Could you check a few things on this model? Use its own coordinates, in mm. Coordinates: 2 decimals unless noted, no trailing zeros. Order: outer loops, then holes, each group sorted by start corner. A loop starts at its lowest first (then second) coordinate and runs counter-clockwise, first axis right, second up. Notation, with made-up numbers: (66, 13.5) -> (107, 13.5) arc R11 ccw to (107, 31.5) -> close; hole circle Ø4 at (-30.75, 69). An arc over 180 degrees is marked (long way). Use a Markdown table: item, result. Add a question column.
1) If I drill on L1, parallel to X at y = 2.2, z = -14; L2, parallel to X at y = 2.75, z = -11.75; L3, parallel to Z at x = -60, y = 2.85, over which ranges is the centre line in solid material (lowest first)? Write a range as [from, to].
2) Will these pins go through, and if not, where does the flat tip stop? pin 1 Ø1.6 at (x, y) = (-59, 1) entering from -Z; pin 2 Ø1.6 at (x, y) = (-65.5, 2) entering from +Z; pin 3 Ø1.5 at (y, z) = (2, 10) entering from -X.
3) If we section it at A-A (y = 2): Write out the boundary of the cut face in (x, z), plus the area to 3 significant figures.
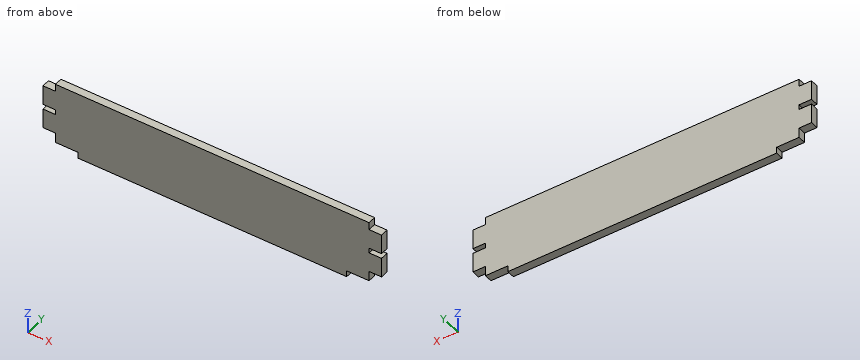
```python
from build123d import *

# Parameters (mm, degrees)
SKETCH1_W               = 5
SKETCH1_H               = 18
SKETCH1_W_2             = 126
SKETCH1_H_2             = 24
SKETCH1_H_3             = 3.5
BOSS_EXTRUDE1_DEPTH     = 3.175
SKETCH2_W               = 9
SKETCH2_H               = 2.5
CUT_EXTRUDE1_DEPTH      = 70.81640656
CUT_EXTRUDE2_DEPTH      = 70.81640656
CUT_EXTRUDE2_DEPTH_BACK = 70.81640656
SKETCH5_W               = 5
SKETCH5_H               = 2


with BuildPart() as part:
    # Sketch1 → Boss-Extrude1 (new body)
    with BuildSketch(Plane(origin=(0, 0, 0), x_dir=(1, 0, 0), z_dir=(0, 1, 0))):
        with Locations((-65.5, 0)):
            Rectangle(SKETCH1_W, SKETCH1_H)
        Rectangle(SKETCH1_W_2, SKETCH1_H_2)
        with Locations((65.5, 0)):
            Rectangle(SKETCH1_W, SKETCH1_H)
        with Locations((0, 13.75)):
            Rectangle(SKETCH1_W_2, SKETCH1_H_3)
    extrude(amount=BOSS_EXTRUDE1_DEPTH)

    # Sketch2 → Cut-Extrude1 (cut, through all)
    with BuildSketch(Plane(origin=(0, 3.175, 0), x_dir=(1, 0, 0), z_dir=(0, 1, 0))):
        with Locations((-58.5, 14.25)):
            Rectangle(SKETCH2_W, SKETCH2_H)
        with Locations((58.5, 14.25)):
            Rectangle(SKETCH2_W, SKETCH2_H)
    extrude(amount=-CUT_EXTRUDE1_DEPTH, mode=Mode.SUBTRACT)

    # Sketch5 → Cut-Extrude2 (cut, two sides: drawn at the far end of the back side and taken through both)
    with BuildSketch(Plane(origin=(0, 3.175, 0), x_dir=(1, 0, 0), z_dir=(0, 1, 0)).offset(-CUT_EXTRUDE2_DEPTH_BACK)):
        with Locations((-65.5, 0)):
            Rectangle(SKETCH5_W, SKETCH5_H)
        with Locations((65.5, 0)):
            Rectangle(SKETCH5_W, SKETCH5_H)
    extrude(amount=CUT_EXTRUDE2_DEPTH + CUT_EXTRUDE2_DEPTH_BACK, mode=Mode.SUBTRACT)


solid = part.part
```
Answer sheet:
| question | item | result |
|---|---|---|
| 1 | L1 | [-54, 54] |
| 1 | L2 | [-63, 63] |
| 1 | L3 | [-13, 12] |
| 2 | pin 1 | z = -13 |
| 2 | pin 2 | z = 9 |
| 2 | pin 3 | x = -63 |
| 3 | outline | (-68, -9) -> (-63, -9) -> (-63, -13) -> (-54, -13) -> (-54, -15.5) -> (54, -15.5) -> (54, -13) -> (63, -13) -> (63, -9) -> (68, -9) -> (68, -1) -> (63, -1) -> (63, 1) -> (68, 1) -> (68, 9) -> (63, 9) -> (63, 12) -> (-63, 12) -> (-63, 9) -> (-68, 9) -> (-68, 1) -> (-63, 1) -> (-63, -1) -> (-68, -1) -> close |
| 3 | area | 3,580 mm2 |
